from build123d import *

# Parameters (mm, degrees)
SKETCH1_R           = 1.5875
SKETCH1_R_2         = 1.25
BOSS_EXTRUDE1_DEPTH = 3


with BuildPart() as part:
    # Sketch1 → Boss-Extrude1 (new body)
    with BuildSketch(Plane.XY):
        with BuildLine():
            Line((-14.954240874, 193.488256671), (-38.94528665, 162.581960817))
            ThreePointArc((-38.94528665, 162.581960817), (-45.259350105, 161.786597572), (-46.05471335, 168.100661026))
            Line((-46.05471335, 168.100661026), (-29.985536617, 188.801664845))
            ThreePointArc((-29.985536617, 188.801664845), (-29.626045817, 190.516785549), (-30.755439529, 191.856689466))
            ThreePointArc((-30.755439529, 191.856689466), (-44.594733066, 194.265558421), (-57.942527266, 189.887763856))
            ThreePointArc((-57.942527266, 189.887763856), (-59.388320452, 189.617207801), (-60.628151377, 190.408622856))
            Line((-60.628151377, 190.408622856), (-63.563416093, 194.467459011))
            ThreePointArc((-63.563416093, 194.467459011), (-63.907898099, 196.011433745), (-63.022949076, 197.322689273))
            ThreePointArc((-63.022949076, 197.322689273), (-60.680350979, 198.710081326), (-58.244425957, 199.926178296))
            Line((-58.244425957, 199.926178296), (-57.415771959, 198.105922118))
            ThreePointArc((-57.415771959, 198.105922118), (-58.320144396, 197.678952012), (-59.212307575, 197.227025207))
            Line((-59.212307575, 197.227025207), (-58.748076809, 196.341310922))
            ThreePointArc((-58.748076809, 196.341310922), (-39.400871452, 200.203832377), (-21.038388075, 192.989081421))
            Line((-21.038388075, 192.989081421), (-20.425199163, 193.779017721))
            ThreePointArc((-20.425199163, 193.779017721), (-21.223653619, 194.381233178), (-22.038528177, 194.961036964))
            Line((-22.038528177, 194.961036964), (-20.333405525, 197.429347468))
            ThreePointArc((-20.333405525, 197.429347468), (-15.617758617, 198.224162104), (-14.954240874, 193.488256671))
        make_face()
        with Locations((-42.5, 165.341310922)):
            Circle(SKETCH1_R, mode=Mode.SUBTRACT)
        with Locations((-17.589064697, 195.53354153)):
            Circle(SKETCH1_R_2, mode=Mode.SUBTRACT)
    extrude(amount=-BOSS_EXTRUDE1_DEPTH)


solid = part.part
The model under review builds one solid part; all positions refer to its coordinate system, in mm. A direction names the side the tool comes from. Round coordinates to 2 decimals unless told otherwise and drop trailing zeros. Loops run counter-clockwise (first coordinate to the right, second up) from the corner with the lowest first, then second, coordinate; pieces in that order, holes last. Notation, with made-up numbers: (88, 66.25) - (94, 66.25) arc R13 cw to (94, 71.25) - close; hole circle Ø10 at (-15.5, -2). An arc over 180 degrees is marked (long way). Use CSV: the item, a comma, the result in double quotes.
(1) The part is to be moulded in two halves that separate along X. For faces 1 (the cylindrical face through (-63.91, 195.99, -1.48)), 2 (the flat face through (-26.782, 178.251, -1.479)), 3 (the flat face through (-33, 184, 0)), 4 (the cylindrical face through (-58.308, 197.685, -1.479)), say which applies: pulls with the +X half, pulls with the -X half, needs draft (parallel to the pull), parting line crosses it, or undercut.
Working result:
face 1,"pulls with the -X half"
face 2,"pulls with the +X half"
face 3,"needs draft"
face 4,"undercut"
(2) Machinability: for faces 5 (the flat face through (-57.836, 199.029, -1.479)), 6 (the flat face through (-38.13, 178.31, -1.48)), 7 (the cylindrical face through (-29.62, 190.49, -1.48)), 8 (the flat face through (-33, 184, -3)), 9 (the cylindrical face through (-60.7, 198.7, -1.5)), which of the approach directions +Z, -Z, +X, -X, +Y, -Y give a long, thin tool a straight path to every point of the face, cutting with its end or side? Answer none if there is none.
Working result:
face 5,"+Z, -Z, +Y"
face 6,"+Z, -Z, -X"
face 7,"+Z, -Z"
face 8,"-Z, +X, -X, +Y, -Y"
face 9,"+Z, -Z, -X, +Y"
(3) Take a section at D-D, the plane y = 172. Give the boundary of the cut face in (x, z), plus the area to 3 significant figures.
Working result:
outline,"(-43.03, -3) - (-31.63, -3) - (-31.63, 0) - (-43.03, 0) - close"
area,"34.2 mm^2"
(4) For line 1 (X direction, y = 197.5, z = -1.05); line 2 (Y direction, x = -42.5, z = -1.3); line 3 (Y direction, x = -43, z = -2.45), list the stretches that pass through material, from the lowest coordinate up.
Working result:
line 1,"x = -62.74 to -58.68, -56.31 to -28.69, -20.28 to -14.89"
line 2,"y = 160.84 to 163.75, 166.93 to 172.68, 194.34 to 200.34"
line 3,"y = 160.87 to 163.83, 166.85 to 172.04, 194.34 to 200.34"
(5) Take a section at B-B, the plane z = -2.05. State how many separate pieces and enclosed holes the cut face has, plus the area to 3 significant figures.
Working result:
separate pieces,"1"
enclosed holes,"2"
area,"616 mm^2"
(6) Clearance check with flat-ended pins moving along their axes: P1, Ø1, axis at x = -38, z = -1.5, coming from the -Y side; P2, Ø1.5, axis at x = -43.5, z = -1.5, coming from the -Y side; P3, Ø1.5, axis at y = 178.5, z = -0.5, coming from the +X side. State where each tip first meets the part, or that it passes through.
Working result:
P1,"stops at y = 163.16"
P2,"stops at y = 160.85"
P3,"stops at x = -26.01"
(7) Take a section at A-A, the plane x = -42.5. Give the boundary of the cut face in (y, z).
Working result:
outline,"(160.84, -3) - (163.75, -3) - (163.75, 0) - (160.84, 0) - close; (166.93, -3) - (172.68, -3) - (172.68, 0) - (166.93, 0) - close; (194.34, -3) - (200.34, -3) - (200.34, 0) - (194.34, 0) - close"
(8) Take a section at C-C, the plane x = -33. Give the boundary of the cut face in (y, z).
Working result:
outline,"(170.24, -3) - (184.92, -3) - (184.92, 0) - (170.24, 0) - close; (192.74, -3) - (199.03, -3) - (199.03, 0) - (192.74, 0) - close"
